Geometry check sheet. Reference: the model listing, model coordinates, mm. A direction names the side the tool comes from. Round coordinates to 2 decimals unless told otherwise and drop trailing zeros. Write each loop counter-clockwise with the first axis right and the second up, starting at its lowest first coordinate (ties: lowest second). Pieces come first, ordered by that corner, then holes. Notation, with made-up numbers: (-16.75, 80.25) -> (-0.75, 80.25) arc R28 cw to (-0.75, 118.25) -> close; hole circle Ø7 at (27.5, 23). An arc over 180 degrees is marked (long way). Return JSON: item names as keys, results as strings. Group by question number.
from build123d import *

# Parameters (mm, degrees)
BOSS_EXTRUDE1_DEPTH = 280
BOSS_EXTRUDE2_START = 140
BOSS_EXTRUDE2_DEPTH = 10


with BuildPart() as part:
    # Sketch1 → Boss-Extrude1 (new body)
    with BuildSketch(Plane(origin=(0, 0, 0), x_dir=(1, 0, 0), z_dir=(0, 1, 0))):
        Polygon((-116.35, -3.175), (-3.175, -3.175), (-3.175, -116.35), (110, -116.35), (110, 110), (-116.35, 110), align=None)
        Polygon((-113.175, 0), (0, 0), (0, -113.175), (106.825, -113.175), (106.825, 106.825), (-113.175, 106.825), align=None, mode=Mode.SUBTRACT)
    extrude(amount=BOSS_EXTRUDE1_DEPTH)

    # Sketch2 → Boss-Extrude2 (add)
    with BuildSketch(Plane(origin=(0, 0, 0), x_dir=(1, 0, 0), z_dir=(0, 1, 0)).offset(BOSS_EXTRUDE2_START)):
        Polygon((-113.175, 106.825), (-113.175, 0), (0, 0), (0, -113.175), (106.825, -113.175), (106.825, 106.825), align=None)
    extrude(amount=BOSS_EXTRUDE2_DEPTH)


solid = part.part
1) Mould release check, pull along Z, two halves, no side actions. Record for faces 6 (the face through (-61, 138, 3.175)), 7 (the face through (-2, 138, -110)), 8 (the face through (-2, 214, -106.825)), 9 (the face through (110, 138, 5)): +Z half, -Z half, draft (parallel to the pull), parting line (faces both ways), or undercut.
2) Sectioned sample at B-B on z = 66. Enter the section's corners in (x, y) (3 decimals), and give its area (3 significant figures).
3) Material ranges on probe 1 along Z at (x, y) = (40, 25.5) (3 decimals); probe 2 along Z at (x, y) = (-48, 191) (3 decimals); probe 3 along X at (y, z) = (58, 53) (3 decimals), recorded low to high. Write a range as [from, to].
4) Sectioned sample at A-A on y = 222. Enter the section's corners in (x, z) (3 decimals), and give its area (3 significant figures).
5) Tool access check on faces 1 (the face through (-116.35, 138, -54)), 2 (the face through (0, 214, 56)), 3 (the face through (-62, 0, 3)), 4 (the face through (-57, 69, 0)), 5 (the face through (-3.175, 138, 59)). Record the directions out of +Z, -Z, +X, -X, +Y, -Y that give a thin tool (end or side, any length) a straight path to the whole face; none if there is none.
6) Sectioned sample at C-C on x = -81.5. Enter the section's corners in (y, z) (3 decimals).
7) Go/stop test with flat-tipped pins: P1, Ø1.5, axis at x = -14, y = 81.5, coming from the +Z side (3 decimals); P2, Ø8, axis at x = -19, z = -78.5, coming from the +Y side. Record where each tip stops, or that it passes through.
Evaluation:
{
 "1": {"face 6": "+Z half", "face 7": "-Z half", "face 8": "undercut", "face 9": "draft"},
 "2": {"outline": "(-3.175, 0) -> (0, 0) -> (0, 140) -> (106.825, 140) -> (106.825, 0) -> (110, 0) -> (110, 280) -> (106.825, 280) -> (106.825, 150) -> (0, 150) -> (0, 280) -> (-3.175, 280) -> close", "area": "2,850 mm2"},
 "3": {"probe 1": "z = [-110, -106.825], [113.175, 116.35]", "probe 2": "z = [-110, -106.825], [0, 3.175]", "probe 3": "x = [-3.175, 0], [106.825, 110]"},
 "4": {"outline": "(-116.35, -110) -> (110, -110) -> (110, 116.35) -> (-3.175, 116.35) -> (-3.175, 3.175) -> (-116.35, 3.175) -> close; hole (-113.175, -106.825) -> (106.825, -106.825) -> (106.825, 113.175) -> (0, 113.175) -> (0, 0) -> (-113.175, 0) -> close", "area": "2,830 mm2"},
 "5": {"face 1": "+Z, -Z, -X, +Y, -Y", "face 2": "+Y", "face 3": "+Z, -Z, +X, -X, -Y", "face 4": "-Y", "face 5": "+Z, -X, +Y, -Y"},
 "6": {"outline": "(0, -110) -> (280, -110) -> (280, -106.825) -> (150, -106.825) -> (150, 0) -> (280, 0) -> (280, 3.175) -> (0, 3.175) -> (0, 0) -> (140, 0) -> (140, -106.825) -> (0, -106.825) -> close"},
 "7": {"P1": "stops at z = 3.175", "P2": "stops at y = 150"}
}
